Read the model definition and answer for the solid it produces. Units are mm, in the model's axes. A direction names the side the tool comes from. Give positions to 0.01 mm unless a question says otherwise; leave off trailing zeros. Write each loop counter-clockwise with the first axis right and the second up, starting at its lowest first coordinate (ties: lowest second). Pieces come first, ordered by that corner, then holes. Notation, with made-up numbers: (-5, 15.25) -> (23, 15.25) arc R18 cw to (23, 37.25) -> close; hole circle Ø2 at (61.25, 39). An arc over 180 degrees is marked (long way). Use a Markdown table: item, result.
from build123d import *

# Parameters (mm, degrees)
SKETCH_1_R      = 15
EXTRUDE_1_DEPTH = 20


with BuildPart() as part:
    # 草圖1 → 填料-伸長1 (new body)
    with BuildSketch(Plane(origin=(0, 0, 0), x_dir=(1, 0, 0), z_dir=(0, 1, 0))):
        with BuildLine():
            Line((0, 30), (-30, 30))
            Line((-30, 30), (-30, 15))
            Line((-30, 15), (-45, 15))
            Line((-45, 15), (-45, 30))
            Line((-45, 30), (-75, 30))
            Line((-75, 30), (-75, -30))
            Line((-75, -30), (-45, -30))
            Line((-45, -30), (-45, -13.222878726))
            Line((-45, -13.222878726), (-30, -13.222878726))
            Line((-30, -13.222878726), (-30, -30))
            Line((-30, -30), (0, -30))
            ThreePointArc((0, -30), (30, 0), (0, 30))
        make_face()
        with Locations(Location((0, 0, 0), (0, 0, 270))):
            Circle(SKETCH_1_R, mode=Mode.SUBTRACT)
    extrude(amount=EXTRUDE_1_DEPTH)


solid = part.part
Item 1: A cutting plane is placed at B-B (z = -20). Give the vertices of the cut face in (x, y), then the cut area to 3 significant figures.
Return value:
| item | result |
|---|---|
| outline | (-75, 0) -> (-45, 0) -> (-45, 20) -> (-75, 20) -> close; (-30, 0) -> (22.36, 0) -> (22.36, 20) -> (-30, 20) -> close |
| area | 1,650 mm^2 |
Item 2: Straight lines are drawn through the part: line 1 along X through (y, z) = (10, 0); line 2 along X through (y, z) = (4, -7). For each, find the intervals that lie inside material, in ascending order. Write a range as [from, to].
Return value:
| item | result |
|---|---|
| line 1 | [-75, -15], [15, 30] |
| line 2 | [-75, -13.27], [13.27, 29.17] |
Item 3: This flat-tipped pin is pushed along its axis until it touches: P1, Ø2, axis at y = 9.5, z = 0, coming from the +X side. Where does it stop, or does it pass through?
Return value:
| item | result |
|---|---|
| P1 | x = 30 |
Item 4: For a pull along Z with two mould halves and no side action, classify faces 1 (the face through (-30, 10, 21)), 2 (the face through (0.66, 9.86, -14.985)), 3 (the face through (-15, 10, 30)) as +Z half, -Z half, draft (parallel to the pull), parting line (faces both ways), or undercut.
Return value:
| item | result |
|---|---|
| face 1 | draft |
| face 2 | undercut |
| face 3 | +Z half |
Item 5: A cutting plane is placed at A-A (y = 5.75). Give the vertices of the cut face in (x, z).
Return value:
| item | result |
|---|---|
| outline | (-75, -30) -> (-45, -30) -> (-45, -15) -> (-30, -15) -> (-30, -30) -> (0, -30) arc R30 ccw to (0, 30) -> (-30, 30) -> (-30, 13.22) -> (-45, 13.22) -> (-45, 30) -> (-75, 30) -> close; hole circle Ø30 at (0, 0) |
Item 6: A tool of negligible diameter and unlimited length cuts with its end or side. For faces 4 (the face through (-45, 10, -22)), 5 (the face through (-45, 10, 22)), 6 (the face through (-75, 10, 0)), from which of +Z, -Z, +X, -X, +Y, -Y can it reach the whole face along a straight path? Write none if from no direction.
Return value:
| item | result |
|---|---|
| face 4 | -Z, +Y, -Y |
| face 5 | +Z, +Y, -Y |
| face 6 | +Z, -Z, -X, +Y, -Y |
Item 7: A cutting plane is placed at C-C (x = -7.5). Give the vertices of the cut face in (y, z), then the cut area to 3 significant figures.
Return value:
| item | result |
|---|---|
| outline | (0, -30) -> (20, -30) -> (20, -12.99) -> (0, -12.99) -> close; (0, 12.99) -> (20, 12.99) -> (20, 30) -> (0, 30) -> close |
| area | 680 mm^2 |
